Can you work these out from the model? Positions are in its coordinate system, mm. A direction names the side the tool comes from. Round coordinates to 2 decimals unless told otherwise and drop trailing zeros. Order: outer loops, then holes, each group sorted by start corner. A loop starts at its lowest first (then second) coordinate and runs counter-clockwise, first axis right, second up. Notation, with made-up numbers: (5, 84) -> (31, 84) arc R17 cw to (31, 88) -> close; hole circle Ø8 at (-21.5, -26.75). An arc over 180 degrees is marked (long way). Use a Markdown table: item, result. Add a question column.
Q1. If we section it at B-B on y = 3.4: List the corners of the cut face in (x, z) for me, plus the area to 3 significant figures.
Q2. I'm going to push flat-ended pins straight in: pin 1 Ø5 at (y, z) = (3.4, 9.35) entering from +X; pin 2 Ø1 at (x, z) = (19, 6) entering from -Y; pin 3 Ø4 at (x, y) = (18.5, 13.5) entering from -Z. Where does each tip first touch, or does it pass through?
Q3. We'd pull the mould along Z, two halves only. Please class faces 3 (the face through (7.1, 12.4, 0)), 4 (the face through (10, 16, 6)), 5 (the face through (0.028, 3.14, 11.333)): +Z half, -Z half, draft (parallel to the pull), parting line (faces both ways), or undercut.
Q4. I need wall thicknesses on line 1 along Z through (x, y) = (-0.6, 3.4); line 2 along Y through (x, z) = (21, 2.75); line 3 along X through (y, z) = (11.5, 1.5). Which ranges of each line are inside material? Lowest first, please. Write a range as [from, to].
Q5. For faces 1 (the face through (2, 6, 6)), 2 (the face through (0.028, 0.301, 11.715)), which set-ups out of +Z, -Z, +X, -X, +Y, -Y let a thin tool reach every point of the face, with its end or its side?
Q6. If we section it at C-C on x = -0.5: List the corners of the cut face in (y, z) for me, plus the area to 3 significant figures.
Autodesk Fusion 360 part; units mm, degrees
sketch "Skizze1" plane through (0, 0, 0) normal (0, 0, 1) x (1, 0, 0)
  line L0 (2, 12) -> (24, 12)
  line L1 (-2, 16) -> (24, 16)
  line L2 (24, 16) -> (24, 12)
  line L3 (2, 0) -> (2, 12)
  line L4 (-2, 0) -> (-2, 16)
  line L5 (-2, 0) -> (2, 0)
extrude "Extrusion1" add sketch "Skizze1" along normal blind 12
sketch "Skizze2" plane through (2, 0, 0) normal (1, 0, 0) x (0, 1, 0)
  line L0 (0, 0) -> (12, 0)
  line L1 (12, 0) -> (12, 12)
  line L2 (12, 12) -> (0, 12)
  line L3 (0, 12) -> (0, 0)
  circle A0 centre (3.4, 9.35) radius 2
  circle A1 centre (3.4, 2.65) radius 2
  dimension "d11" = 4
  dimension "d13" = 4
extrude "Extrusion2" cut sketch "Skizze2" against normal blind 12 contours A0 | A1
fillet "Abrundung1" radius 2 2 edges at (24, 16, 6) (24, 12, 6)
fillet "Abrundung2" radius 1 2 edges at (0, 0, 12) (0, 0, 0)
Answer below:
| question | item | result |
|---|---|---|
| 1 | outline | (-2, 0) -> (2, 0) -> (2, 0.65) -> (-2, 0.65) -> close; (-2, 4.65) -> (2, 4.65) -> (2, 7.35) -> (-2, 7.35) -> close; (-2, 11.35) -> (2, 11.35) -> (2, 12) -> (-2, 12) -> close |
| 1 | area | 16.0 mm² |
| 2 | pin 1 | x = 2 |
| 2 | pin 2 | y = 12 |
| 2 | pin 3 | z = 0 |
| 3 | face 3 | -Z half |
| 3 | face 4 | draft |
| 3 | face 5 | undercut |
| 4 | line 1 | [0, 0.65], [4.65, 7.35], [11.35, 12] |
| 4 | line 2 | [12, 16] |
| 4 | line 3 | [-2, 2] |
| 5 | face 1 | +Z, -Z, +X, -Y |
| 5 | face 2 | +Z, +X, -X, -Y |
| 6 | outline | (0, 1) arc R1 ccw to (1, 0) -> (16, 0) -> (16, 12) -> (1, 12) arc R1 ccw to (0, 11) -> close; hole circle Ø4 at (3.4, 2.65); hole circle Ø4 at (3.4, 9.35) |
| 6 | area | 166 mm² |
